Check sheet for the modelled part. Datum: model origin and axes. Units: mm. A direction names the side the tool comes from. Coordinates: 2 decimals unless noted, no trailing zeros. Loops run counter-clockwise (first coordinate to the right, second up) from the corner with the lowest first, then second, coordinate; pieces in that order, holes last. Notation, with made-up numbers: (59, -25) -> (74, -25) arc R28 ccw to (74, 2) -> close; hole circle Ø2 at (5.25, 16). An arc over 180 degrees is marked (long way). Use CSV: the item, a comma, the result in double quotes. Start each with the question number.
1. Sectioned sample at C-C, the plane y = 6. Record the cut outline in (x, z), and give its area (3 significant figures).
2. Sectioned sample at B-B, the plane x = 23. Record the cut outline in (y, z).
3. Gauge pin test, flat ends, axial feed: pin 1 (2 mm diameter, centred on y = 4, z = -46.5, fed in from +X); pin 2 (1.2 mm diameter, centred on y = 11, z = -56, fed in from -X); pin 3 (2 mm diameter, centred on x = 52, y = 2, fed in from -Z); pin 4 (5 mm diameter, centred on y = -15.5, z = -42.5, fed in from +X). Record the tip position at first contact, or that the pin passes through.
4. Thickness scan on L1, parallel to Y at x = 42, z = -21; L2, parallel to Z at x = 10.5, y = 7; L3, parallel to X at y = 7, z = -15. Record the ranges inside material, lowest first.
5. Set-up check for faces 1 (the face through (22, 8, -56.584)), 2 (the face through (32.4, 14.43, -57.54)), 3 (the face through (27.5, -5, -25)), 4 (the face through (44.452, -20.796, -14.566)), 5 (the face through (25, 5, -26)): record each of +Z, -Z, +X, -X, +Y, -Y from which the full face is reachable in a straight line by a thin tool's end or side.
6. Sectioned sample at D-D, the plane x = 48. Record the cut outline in (y, z), and give its area (4 significant figures).
7. Sectioned sample at A-A, the plane z = -37. Record the cut outline in (x, y).
8. Release check for a two-part mould opening along Z. For faces 6 (the face through (25, 9, -5)), 7 (the face through (51, 4, -24.5)), 8 (the face through (17.5, 8, -56)), 9 (the face through (33, 10, -57)) record: pulls with the +Z half, pulls with the -Z half, needs draft (parallel to the pull), parting line crosses it, or undercut.
Autodesk Inventor part; units mm, degrees
ref_plane "Work Plane2" through (42.5, -25, -25) normal (0, -1, 0) x (1, 0, 0)
ref_plane "YZ Plane" through (0, 0, 0) normal (1, 0, 0) x (0, 1, 0)
ref_plane "XZ Plane" through (0, 0, 0) normal (0, 1, 0) x (-1, 0, 0)
sketch "Sketch1" plane through (0, 0, 0) normal (0, 1, 0) x (-1, 0, 0)
  line L0 (0, 0) -> (0, -60)
  line L1 (0, 0) -> (-50, 0)
  line L2 (-5, -60) -> (-5, -5)
  line L3 (-5, -5) -> (-50, -5)
  line L4 (-47.5, 69.0442) -> (-47.5, -71.5611) construction
  line L5 (-50, 0) -> (-55, 0)
  line L6 (-55, 0) -> (-55, -50)
  line L7 (-55, -50) -> (-75, -50)
  line L8 (-75, -50) -> (-75, -60)
  line L9 (-75, -60) -> (-45, -60)
  line L10 (-5, -60) -> (-21, -60)
  circle A0 centre (-47.5, -73.124) radius 8.5
  line L11 (16.7028, -43.5) -> (-102.7124, -43.5) construction
  line L12 (-45, -26.5) -> (-50, -26.5)
  line L13 (-50, -26.5) -> (-50, -60.5)
  line L14 (-50, -60.5) -> (-45, -60.5)
  line L15 (-45, -60.5) -> (-45, -26.5)
  line L16 (-45, -43.5) -> (-50, -43.5) construction
  line L17 (-21, -60) -> (-21, -67.124)
  line L18 (-21, -67.124) -> (-30, -67.124)
  line L19 (-39, -67.124) -> (-39, -60)
  line L20 (-39, -60) -> (-45, -60) construction
  line L21 (-15.952, -100.4576) -> (-35.952, -100.4576)
  line L22 (-35.952, -108.4576) -> (-15.952, -108.4576)
  line L23 (-15.952, -108.4576) -> (-15.952, -100.4576)
  line L24 (-15.952, -73.124) -> (-76.4965, -73.124) construction
  line L25 (-30, -57.9879) -> (-30, -83.8601) construction
  line L26 (-25.952, -100.4576) -> (-25.952, -108.4576) construction
  line L27 (-45, -31) -> (-50, -31) construction
  line L28 (-50, -31) -> (-50, -56)
  line L29 (-50, -56) -> (-45, -56) construction
  line L30 (-45, -56) -> (-45, -31)
  line L31 (-45, -56) -> (-50, -56)
  line L32 (-45, -65.1391) -> (-45, -56)
  line L33 (-45, -56) -> (-50, -56)
  line L34 (-50, -56) -> (-50, -65)
  line L35 (-50, -65) -> (-45, -65)
  line L36 (-45, -65) -> (-45, -56)
  arc A1 (-35.952, -108.4576) -> (-35.952, -100.4576) centre (-43.452, -104.4576) ccw
  line L37 (-30, -67.124) -> (-39, -67.124)
  point P0 (-47.5, -43.5)
  point P1 (-30, -73.124)
  dimension "d9" = 17
  dimension "d0" = 60
  dimension "d1" = 50
  dimension "d2" = 5
  dimension "d3" = 47.5
  dimension "d4" = 5
  dimension "d5" = 50
  dimension "d6" = 20
  dimension "d7" = 30
  dimension "d10" = 38.5
  dimension "d11" = 5
  dimension "d12" = 34
  dimension "d13" = 20
  dimension "d14" = 8
  dimension "d57" = 25
  dimension "d58" = 4.5
  dimension "d59" = 5
  dimension "d60" = 9
  dimension "d61" = 17
  dimension "d62" = 9
  dimension "d63" = 9
  dimension "d64" = 9
  dimension "d65" = 6
sketch "Sketch2" plane through (0, 0, 0) normal (0, 1, 0) x (-1, 0, 0)
  line L0 (0, 0) -> (-45, 0)
  line L1 (-45, -60) -> (0, -60)
  line L2 (0, -60) -> (0, 0)
  line L3 (-5, -60) -> (-21, -60)
  line L4 (-30, -67.124) -> (-39, -67.124)
  line L5 (-57.5, -67.124) -> (-72, -67.124)
  line L6 (-72, -67.124) -> (-72, -59.124)
  line L7 (-72, -59.124) -> (-60, -59.124)
  line L8 (-60, -59.124) -> (-60, 0)
  line L9 (-57.5, -67.124) -> (-57.5, -60)
  line L10 (-45, -60.5) -> (-45, -26.5)
  line L11 (-45, -60) -> (-45, 0)
  point P0 (-60, -55)
  point P1 (-60, -67.124)
  dimension "d16" = 57.5
  dimension "d73" = 8
extrude "Extrusion1" add sketch "Sketch2" along normal blind 15
sketch "Sketch3" plane through (0, 15, 0) normal (0, 1, 0) x (1, 0, 0)
  line L0 (5, 5) -> (55, 5)
  line L1 (55, 5) -> (55, 55)
  line L2 (55, 55) -> (5, 55)
  line L3 (5, 55) -> (5, 5)
  line L4 (0, 0) -> (45, 0)
  line L5 (0, 60) -> (0, 0)
  point P0 (60, 0)
  dimension "d23" = 5
  dimension "d24" = 5
  dimension "d25" = 50
  dimension "d26" = 50
extrude "Extrusion2" cut sketch "Sketch3" against normal blind 10
sketch "Sketch5" plane through (0, 0, 0) normal (0, -1, 0) x (1, 0, 0)
  line L0 (45, -60) -> (0, -60)
  line L1 (45, -60.5) -> (45, -26.5)
  line L2 (5, -60) -> (5, -5)
  line L3 (50, -26.5) -> (50, -60.5)
  line L4 (45, -26.5) -> (50, -26.5)
  line L5 (50, -60.5) -> (45, -60.5)
  line L6 (52, -60) -> (52, -24.5)
  line L7 (52, -24.5) -> (43, -24.5)
  line L8 (43, -24.5) -> (43, -60)
  line L9 (52, -60.5) -> (52, -60)
  line L10 (52, -60) -> (43, -60)
  point P0 (80, -60)
  point P1 (57.5, -60)
  dimension "d30" = 40
  dimension "d31" = 2
extrude "Extrusion3" cut sketch "Sketch5" against normal through all contours L0 L8 L7 L6 L10 L3 L4 L1 | L1 L4 L3 L10
sketch "Sketch8" plane through (0, 5, 0) normal (0, 1, 0) x (1, 0, 0)
  line L0 (36, 11.5) -> (39, 11.5)
  line L1 (39, 11.5) -> (39, 43.5)
  line L2 (39, 43.5) -> (36, 43.5)
  line L3 (36, 43.5) -> (36, 11.5)
  line L4 (45, 60.5) -> (45, 26.5)
  line L5 (-16.7028, 43.5) -> (102.7124, 43.5) construction
  point P0 (0, 0)
  point P1 (47.5, 43.5)
  dimension "d45" = 6
  dimension "d46" = 32
  dimension "d47" = 3
extrude "Extrusion5" [suppressed]
sketch "Sketch9" plane through (0, 5, 0) normal (0, 1, 0) x (1, 0, 0)
  line L0 (36, 43.5) -> (39, 43.5)
  line L1 (5, 5) -> (5, 55)
  line L2 (8, 18.5) -> (5, 18.5)
  line L3 (5, 18.5) -> (5, 38.5)
  line L4 (5, 38.5) -> (8, 38.5)
  line L5 (8, 38.5) -> (8, 18.5)
  point P0 (0, 0)
  dimension "d50" = 3
  dimension "d51" = 5
  dimension "d52" = 20
extrude "Extrusion6" add sketch "Sketch9" along normal up to surface (10 mm away)
fillet "Fillet1" radius 0.6 4 edges at (5, 10, -38.5) (8, 10, -38.5) (8, 10, -18.5) (5, 10, -18.5)
fillet "Fillet2" radius 1 1 edges at (43, 2.5, -24.5)
sketch "Sketch15" plane through (0, 0, 0) normal (0, -1, 0) x (1, 0, 0)
  line L0 (0, 0) -> (45, 0)
  line L1 (27.5, 0) -> (57.5, 0)
  line L2 (57.5, 0) -> (57.5, -50)
  line L3 (57.5, -50) -> (27.5, -50)
  line L4 (27.5, -50) -> (27.5, 0)
  line L5 (42.5, -50) -> (42.5, 0) construction
  line L6 (47.5, 69.0442) -> (47.5, -71.5611) construction
  line L7 (0, -60) -> (0, 0)
  dimension "d87" = 30
  dimension "d90" = 50
  dimension "d127" = 27.5
extrude "Extrusion11" add sketch "Sketch15" along normal blind 10
sketch "Sketch17" plane through (45, 5, -5) normal (1, 0, 0) x (0, 0, -1)
  line L0 (-5, -5) -> (-5, 10)
  line L1 (-5, -5) -> (19.5, -5)
  line L2 (-5, 2.5) -> (19.5, 2.5)
  line L3 (19.5, 2.5) -> (19.5, -5)
  line L4 (19.5, -5) -> (-5, -5)
  line L5 (-5, -5) -> (-5, 2.5)
extrude "Extrusion13" add sketch "Sketch17" along normal up to surface (12.5 mm away)
sketch "Sketch18" plane through (0, -10, 0) normal (0, -1, 0) x (1, 0, 0)
  line L0 (27.5, -50) -> (57.5, -50)
  line L1 (57.5, 0) -> (27.5, 0)
  line L2 (42.5, 0) -> (42.5, -50) construction
  line L3 (43, -50) -> (57.5, -50)
  line L4 (57.5, 0) -> (49.5, 0)
  line L5 (49.5, 0) -> (49.5, -50)
  line L6 (49.5, -50) -> (57.5, -50)
  line L7 (57.5, -50) -> (57.5, 0)
  point P0 (0, 0)
  dimension "d95" = 7
revolve "Revolution1" add sketch "Sketch18" angle 180 about axis through (42.5, -10, 0) along (0, 0, -1)
hole "Hole2" at (42.5, -10, 0) direction (0, 0, -1) diameter 14 end through all
ref_plane "Work Plane2" through (42.5, -25, -25) normal (0, -1, 0) x (1, 0, 0)
sketch "Sketch19" plane through (42.5, -25, -25) normal (0, -1, 0) x (1, 0, 0)
  line L0 (-15, 25) -> (-15, -25)
  line L1 (15, -25) -> (-15, -25)
  line L2 (15, -25) -> (15, 25)
  line L3 (15, 25) -> (-15, 25)
  line L4 (0, 10) -> (-15, 10)
  line L5 (-15, -25) -> (-15, 25)
  line L6 (0, 10) -> (15, 10)
  point P0 (-42.5, 25)
  dimension "d106" = 15
hole "Hole3" at (42.5, -25, -15) direction (0, 1, 0) diameter 4 end up to surface
sketch "Sketch20" plane through (43, 0, -60) normal (1, 0, 0) x (0, 0, -1)
  line L0 (-34.5, 0) -> (-34.5, 5)
  line L1 (-10, 0) -> (-34.5, 0)
  line L2 (0, 0) -> (-34.5, 0)
  line L3 (0, 15) -> (0, 0)
  line L4 (-5, 15) -> (0, 15)
  line L5 (-5, 5) -> (-5, 15)
  line L6 (-34.5, 5) -> (-5, 5)
  line L7 (-10, -3) -> (-10, -17)
  line L8 (-10, -10) -> (-60, -10)
  line L9 (-5, 5) -> (-55, 5)
  line L10 (-55, 5) -> (-55, 31)
  line L11 (-55, 31) -> (-5, 31)
  line L12 (-5, 31) -> (-5, 5)
  circle A0 centre (-16, 23) radius 11
  circle A1 centre (-16, 23) radius 18
  point P0 (-60, 0)
  dimension "d114" = 50
  dimension "d115" = 26
  dimension "d116" = 22
  dimension "d117" = 33
  dimension "d129" = 36
sketch "Sketch21" plane through (43, 0, -60) normal (1, 0, 0) x (0, 0, -1)
  line L0 (-5, 15) -> (0, 15)
  line L1 (-5, 5) -> (-5, 15)
  line L2 (-20.9, 5) -> (-5, 5)
  line L3 (0, 5) -> (0, 15)
  line L4 (0, 15) -> (-5, 15)
  line L5 (-5, 15) -> (-5, 5)
  line L6 (-5, 5) -> (0, 5)
  point P0 (-60, 0)
extrude "Extrusion14" cut sketch "Sketch21" against normal blind 10
fillet "Fillet3" radius 2 2 edges at (33, 5, -57.5) (33, 15, -57.5)
sketch "Sketch22" plane through (0, 5, 0) normal (0, 1, 0) x (1, 0, 0)
  line L0 (35, 55) -> (35, 60)
  line L1 (5, 55) -> (35, 55)
  line L2 (5, 39.1) -> (5, 55)
  arc A0 (5, 39.1) -> (5.6, 38.5) centre (5.6, 39.1) ccw
  line L3 (5.6, 38.5) -> (7.4, 38.5)
  arc A1 (8, 37.9) -> (7.4, 38.5) centre (7.4, 37.9) ccw
  line L4 (8, 37.9) -> (8, 19.1)
  arc A2 (7.4, 18.5) -> (8, 19.1) centre (7.4, 19.1) ccw
  line L5 (7.4, 18.5) -> (5.6, 18.5)
  arc A3 (5.6, 18.5) -> (5, 17.9) centre (5.6, 17.9) ccw
  line L6 (5, 5) -> (5, 17.9)
  line L7 (45, 5) -> (5, 5)
  line L8 (45, 0) -> (45, 5)
  line L9 (45, 0) -> (57.5, 0)
  line L10 (57.5, 0) -> (57.5, 24.5)
  line L11 (57.5, 24.5) -> (44, 24.5)
  arc A4 (43, 25.5) -> (44, 24.5) centre (44, 25.5) ccw
  line L12 (43, 60) -> (43, 25.5)
  line L13 (35, 60) -> (43, 60)
  line L14 (39, 43.5) -> (39, 11.5)
  line L15 (39, 11.5) -> (36, 11.5)
  line L16 (36, 11.5) -> (36, 43.5)
  line L17 (36, 43.5) -> (39, 43.5)
  line L18 (49.5, 0) -> (35.5, 0)
  line L19 (35.5, 50) -> (49.5, 50)
  line L20 (35.5, 50) -> (49.5, 50)
  line L21 (57.5, 50) -> (27.5, 50)
  line L22 (43, 50) -> (27.5, 50)
  line L23 (43, 50) -> (57.5, 50)
  line L24 (35.5, 50) -> (49.5, 50)
  line L25 (42.5, 50) -> (42.5, 0) construction
  line L26 (49.5, 0) -> (35.5, 0)
  line L27 (5, 55) -> (45, 55)
  line L28 (45, 55) -> (45, 5)
  line L29 (45, 5) -> (5, 5)
  line L30 (5, 5) -> (5, 55)
  line L31 (45, 55) -> (51, 55)
  line L32 (51, 55) -> (51, 33)
  line L33 (51, 33) -> (45, 33)
  line L34 (45, 33) -> (45, 55)
  line L35 (48, 55) -> (48, 33) construction
  point P0 (0, 0)
  point P1 (45, 24.5)
  dimension "d121" = 40
  dimension "d122" = 50
  dimension "d123" = 40
  dimension "d124" = 6
  dimension "d125" = 22
  dimension "d128" = 5.5
sketch "Sketch23" plane through (0, 15, 0) normal (0, 1, 0) x (1, 0, 0)
  line L0 (45, 5) -> (5, 5)
  line L1 (33, 55) -> (31, 55)
  line L2 (26, 6.5) -> (17.5, 6.5)
  line L3 (17.5, 6.5) -> (17.5, 5)
  line L4 (17.5, 5) -> (26, 5)
  line L5 (26, 5) -> (26, 6.5)
  line L6 (31, 60) -> (31, 55)
  line L7 (17.5, 56.5837) -> (26, 56.5837)
  line L8 (26, 56.5837) -> (26, 55.0837)
  line L9 (26, 55.0837) -> (17.5, 55.0837)
  line L10 (17.5, 55.0837) -> (17.5, 56.5837)
  dimension "d131" = 1.5
  dimension "d134" = 8.5
  dimension "d135" = 1.5
  dimension "d136" = 5
  dimension "d137" = 8.5
extrude "Extrusion15" cut sketch "Sketch23" against normal through all
properties part number "HousingV2"
Completed:
1,outline,"(0, -60) -> (33.27, -60) -> (33.27, -55) -> (5, -55) -> (5, -39.1) arc R0.6 cw to (5.6, -38.5) -> (7.4, -38.5) arc R0.6 ccw to (8, -37.9) -> (8, -19.1) arc R0.6 ccw to (7.4, -18.5) -> (5.6, -18.5) arc R0.6 cw to (5, -17.9) -> (5, -5) -> (45, -5) -> (45, -24.5) -> (57.5, -24.5) -> (57.5, 0) -> (0, 0) -> close; hole (17.5, -56.58) -> (26, -56.58) -> (26, -55.08) -> (17.5, -55.08) -> close"
1,area,"995 mm²"
2,outline,"(0, -60) -> (15, -60) -> (15, -56.58) -> (0, -56.58) -> close; (0, -55.08) -> (15, -55.08) -> (15, -55) -> (5, -55) -> (5, -6.5) -> (0, -6.5) -> close; (0, -5) -> (15, -5) -> (15, 0) -> (0, 0) -> close"
3,pin 1,"x = 43"
3,pin 2,"x = 0"
3,pin 3,"z = -24.5"
3,pin 4,"x = 57.2"
4,L1,"-24.99 to -16.98, -3.02 to 5"
4,L2,"-60 to -55, -5 to 0"
4,L3,"0 to 5, 45 to 57.5"
5,face 1,"+Y, -Y"
5,face 2,"-Z, +X, +Y"
5,face 3,"+Z, -Z, -X, -Y"
5,face 4,"-Y"
5,face 5,"+Y"
6,outline,"(-23.96, -50) -> (-14.33, -50) -> (-14.33, 0) -> (-23.96, 0) -> close; (-5.67, -50) -> (0, -50) -> (0, -24.5) -> (7.5, -24.5) -> (7.5, 0) -> (-5.67, 0) -> close"
6,area,"948.5 mm²"
7,outline,"(0, 0) -> (27.5, 0) -> (27.5, -10) arc R15 ccw to (57.5, -10) -> (57.5, 0) -> (43, 0) -> (43, 5) -> (8, 5) -> (8, 15) -> (0, 15) -> close; hole circle Ø14 at (42.5, -10)"
8,face 6,"undercut"
8,face 7,"pulls with the -Z half"
8,face 8,"undercut"
8,face 9,"needs draft"
